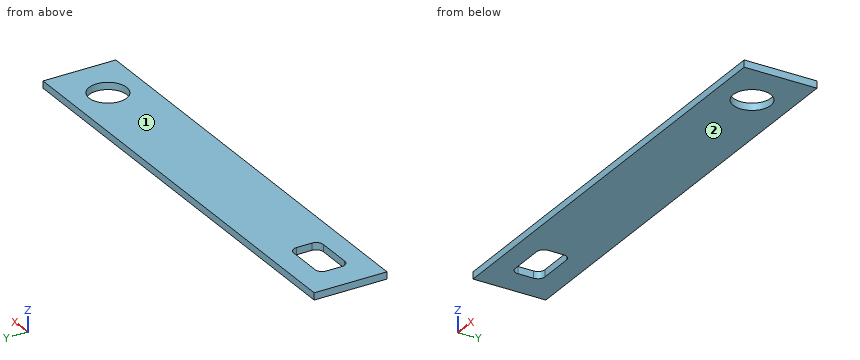
```python
from build123d import *

# Parameters (mm, degrees)
SKETCH1_W          = 190
SKETCH1_H          = 31
SKETCH1_R          = 8
BASE_FLANGE1_DEPTH = 3


# Sheet-metal steps are written as plain solids
with BuildPart() as part:
    # Sketch1 → Base-Flange1 (new body)
    with BuildSketch(Plane.XY):
        with Locations((95, 15.5)):
            Rectangle(SKETCH1_W, SKETCH1_H)
        with Locations((170, 15.5)):
            Circle(SKETCH1_R, mode=Mode.SUBTRACT)
        with BuildLine():
            Line((15, 21.5), (30, 21.5))
            ThreePointArc((30, 21.5), (32.121320344, 20.621320344), (33, 18.5))
            Line((33, 18.5), (33, 11.9))
            ThreePointArc((33, 11.9), (32.121320344, 9.778679656), (30, 8.9))
            Line((30, 8.9), (15, 8.9))
            ThreePointArc((15, 8.9), (12.878679656, 9.778679656), (12, 11.9))
            Line((12, 11.9), (12, 18.5))
            ThreePointArc((12, 18.5), (12.878679656, 20.621320344), (15, 21.5))
        make_face(mode=Mode.SUBTRACT)
    extrude(amount=-BASE_FLANGE1_DEPTH)


solid = part.part
```
Build history of the part. All positions in model axes, mm. Face numbers are marked on the shaded views. Give positions to 0.01 mm unless a question says otherwise; leave off trailing zeros. Loops run counter-clockwise (first coordinate to the right, second up) from the corner with the lowest first, then second, coordinate; pieces in that order, holes last.
1) Two-plate mould, pull along Z, no slides. Class the marked faces 1 and 2: released by +Z, released by -Z, zero draft, split by the parting line, or undercut.
Values follow:
face 1: released by +Z
face 2: released by -Z
2) Drop flat-ended pins along their axis: P1, Ø9.5, axis at x = 170, y = 15.5, coming from the -Z side; P2, Ø1, axis at x = 160.5, y = 17, coming from the +Z side. Give the stop position or say it passes through.
Values follow:
P1: passes through
P2: stops at z = 0
3) Band-saw the part on D-D on x = 170. List the corners of the cut face in (y, z).
Values follow:
outline: (0, -3) - (7.5, -3) - (7.5, 0) - (0, 0) - close; (23.5, -3) - (31, -3) - (31, 0) - (23.5, 0) - close
4) Band-saw the part on A-A on x = 25.5. List the corners of the cut face in (y, z).
Values follow:
outline: (0, -3) - (8.9, -3) - (8.9, 0) - (0, 0) - close; (21.5, -3) - (31, -3) - (31, 0) - (21.5, 0) - close
5) Probe line 1 along X through (y, z) = (15, -1.6); line 2 along X through (y, z) = (14, -1.7); line 3 along Y through (x, z) = (19.5, -1.1). List the from-to ranges inside material, lowest first.
Values follow:
line 1: x = 0 to 12, 33 to 162.02, 177.98 to 190
line 2: x = 0 to 12, 33 to 162.14, 177.86 to 190
line 3: y = 0 to 8.9, 21.5 to 31
6) Band-saw the part on C-C on y = 15.5. List the corners of the cut face in (x, z).
Values follow:
outline: (0, -3) - (12, -3) - (12, 0) - (0, 0) - close; (33, -3) - (162, -3) - (162, 0) - (33, 0) - close; (178, -3) - (190, -3) - (190, 0) - (178, 0) - close
7) Band-saw the part on B-B on z = -2.4. List the corners of the cut face in (x, y), then the cut area to 3 significant figures.
Values follow:
outline: (0, 0) - (190, 0) - (190, 31) - (0, 31) - close; hole (12, 11.9) arc R3 ccw to (15, 8.9) - (30, 8.9) arc R3 ccw to (33, 11.9) - (33, 18.5) arc R3 ccw to (30, 21.5) - (15, 21.5) arc R3 ccw to (12, 18.5) - close; hole circle Ø16 at (170, 15.5)
area: 5,430 mm2
